Can you work these out from the model? Positions are in its coordinate system, mm. Face numbers are marked on the shaded views. A direction names the side the tool comes from. Round coordinates to 2 decimals unless told otherwise and drop trailing zeros. Order: outer loops, then holes, each group sorted by start corner. A loop starts at its lowest first (then second) coordinate and runs counter-clockwise, first axis right, second up. Notation, with made-up numbers: M 68,50 L 90,50 A5 ccw 90,54 Z; hole C -16,52.25 d9. An arc over 180 degrees is marked long. One line per question, with ' | ' between items.
```python
from build123d import *

# Parameters (mm, degrees)
F0_W     = 127
F0_H     = 152.4
F1_DEPTH = 50.8
F2_W     = 127
F2_H     = 50.8
F3_DEPTH = 76.2
F4_W     = 127
F4_H     = 50.8
F5_DEPTH = 101.6
F6_W     = 50.8
F6_H     = 76.2
F7_DEPTH = 101.6


with BuildPart() as f1:
    # F0 (on Front) → F1 (new body)
    with BuildSketch(Plane.XZ):
        with Locations((4.05114, 7.757214)):
            Rectangle(F0_W, F0_H)
    extrude(amount=F1_DEPTH)

    # F2 (on face) → F3 (join)
    with BuildSketch(Plane(origin=(0, 0, 0), x_dir=(-1, 0, 0), z_dir=(0, 1, 0))):
        with Locations((-4.05114, 58.557214)):
            Rectangle(F2_W, F2_H)
    extrude(amount=F3_DEPTH)

    # F4 (on face) → F5 (join)
    with BuildSketch(Plane.XZ.offset(50.8)):
        with Locations((4.05114, -43.042786)):
            Rectangle(F4_W, F4_H)
    extrude(amount=F5_DEPTH)

    # F6 (on face) → F7 (join)
    with BuildSketch(Plane.XY.offset(-17.642786)):
        with Locations((42.15114, -88.9)):
            Rectangle(F6_W, F6_H)
    extrude(amount=F7_DEPTH)


solid = f1.part
```
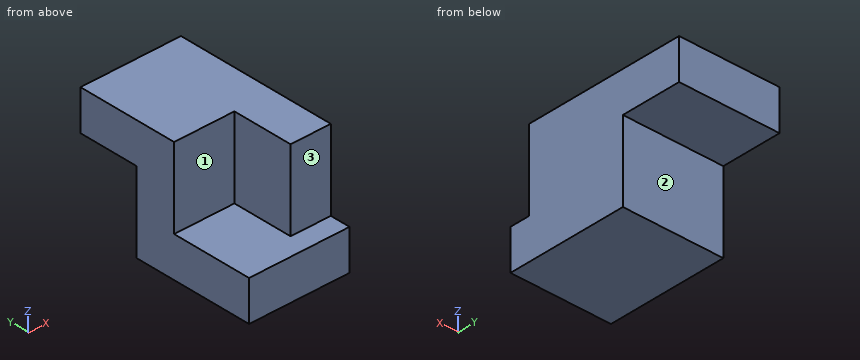
(1) If we section it at A-A on x = 28.5: Please give me the cut outline in (y, z), plus the area to 3 significant figures.
Final values:
outline: M -152.4,-68.44 L 0,-68.44 L 0,33.16 L 76.2,33.16 L 76.2,83.96 L -127,83.96 L -127,-17.64 L -152.4,-17.64 Z | area: 24,500 mm^2
(2) If we section it at B-B on y = -93: Please give me the cut outline in (x, z).
Final values:
outline: M -59.45,-68.44 L 67.55,-68.44 L 67.55,83.96 L 16.75,83.96 L 16.75,-17.64 L -59.45,-17.64 Z
(3) On a 3-axis mill with a long thin cutter (end or side, diameter ignored), from which of +Z, -Z, +X, -X, +Y, -Y can I reach the whole of each face in a straight line? I mean the marked faces 1, 2 and 3. Say none if no direction works.
Final values:
face 1: +Z, -X, -Y | face 2: -Z, +X, -X, +Y | face 3: +Z, +X, -X, -Y
(4) Will these pins go through, and if not, where does the flat tip stop? pin 1 Ø6 at (x, z) = (26, 4) entering from +Y; pin 2 Ø23 at (x, z) = (-11, 55) entering from -Y; pin 3 Ø2 at (x, z) = (47.5, 14) entering from -Y.
Final values:
pin 1: y = 0 | pin 2: y = -50.8 | pin 3: y = -127
(5) If we section it at D-D on x = -18.5: Please give me the cut outline in (y, z), plus the area to 3 significant figures.
Final values:
outline: M -152.4,-68.44 L 0,-68.44 L 0,33.16 L 76.2,33.16 L 76.2,83.96 L -50.8,83.96 L -50.8,-17.64 L -152.4,-17.64 Z | area: 16,800 mm^2
(6) Please list where these lines run through material, in increasing order: probe 1 along Z at (x, y) = (-45, 48); probe 2 along Y at (x, z) = (27.5, -20); probe 3 along Y at (x, z) = (-50.5, 77.5). Write a range as [from, to].
Final values:
probe 1: [33.16, 83.96] | probe 2: [-152.4, 0] | probe 3: [-50.8, 76.2]
(7) If we section it at C-C on z = -4: Please give me the cut outline in (x, y), plus the area to 3 significant figures.
Final values:
outline: M -59.45,-50.8 L 16.75,-50.8 L 16.75,-127 L 67.55,-127 L 67.55,0 L -59.45,0 Z | area: 10,300 mm^2
